The figure shows three views and two pictorial views of one solid part (mm, origin at its lowest corner). Answer the questions. Give positions to 0.01 mm unless a question says otherwise; leave off trailing zeros. Order: outer loops, then holes, each group sorted by start corner. A loop starts at its lowest first (then second) coordinate and runs counter-clockwise, first axis right, second up. Notation, with made-up numbers: (14.25, 35.5) -> (19.25, 35.5) arc R22 cw to (19.25, 45.5) -> close; hole circle Ø4 at (62, 29). An arc over 180 degrees is marked (long way). Use one line per item in the form item = value.
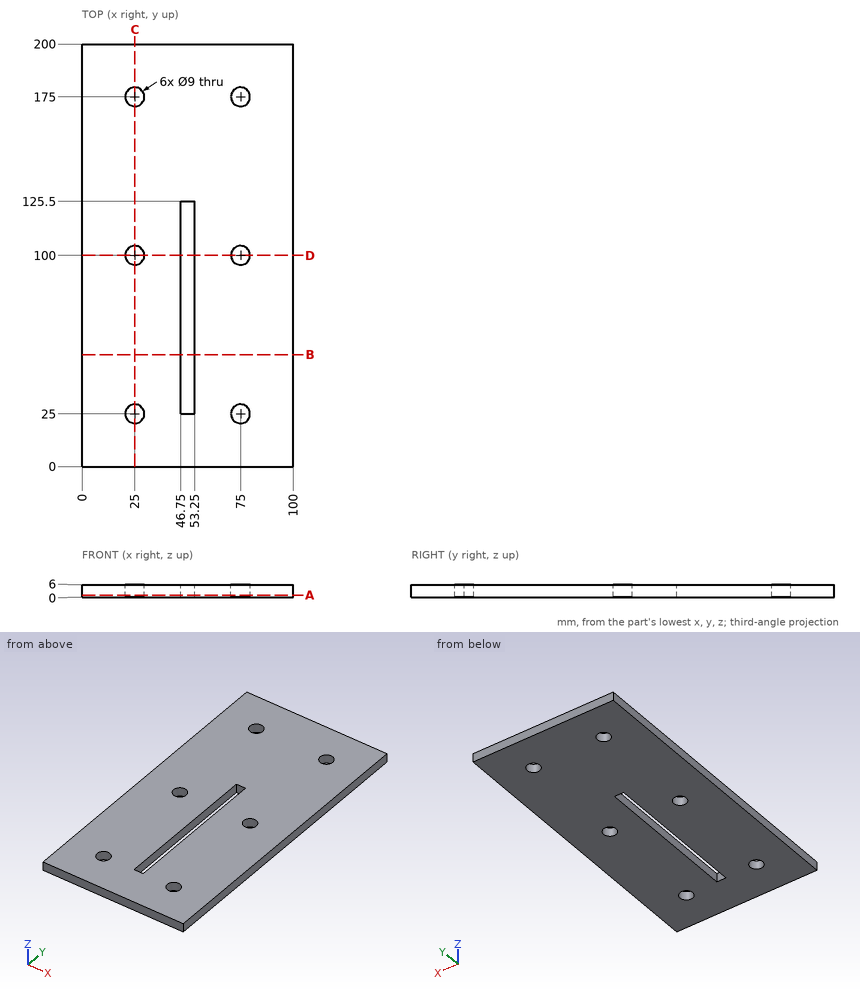
Item 1: The part is cut by section A-A on z = 1. Give the vertices of the cut face in (x, y), and give its area (3 significant figures).
Checks:
outline = (0, 0) -> (100, 0) -> (100, 200) -> (0, 200) -> close; hole circle Ø9 at (25, 25); hole circle Ø9 at (25, 100); hole circle Ø9 at (25, 175); hole (46.75, 25) -> (53.25, 25) -> (53.25, 125.5) -> (46.75, 125.5) -> close; hole circle Ø9 at (75, 25); hole circle Ø9 at (75, 100); hole circle Ø9 at (75, 175)
area = 19,000 mm²
Item 2: Given pin 1 Ø5.5 at (x, y) = (25, 25) entering from +Z, flat-ended and moving along its own axis, determine where the tip first touches the part or whether it passes through.
Checks:
pin_1 = through
Item 3: Straight lines are drawn through the part: L1, parallel to Y at x = 75, z = 2.1; L2, parallel to X at y = 100, z = 2; L3, parallel to X at y = 50.5, z = 3.2. For each, find the intervals that lie inside material, in ascending order. Write a range as from..to.
Checks:
L1 = 0..20.5, 29.5..95.5, 104.5..170.5, 179.5..200
L2 = 0..20.5, 29.5..46.75, 53.25..70.5, 79.5..100
L3 = 0..46.75, 53.25..100
Item 4: The part is cut by section C-C on x = 25. Give the vertices of the cut face in (y, z), and give its area (3 significant figures).
Checks:
outline = (0, 0) -> (20.5, 0) -> (20.5, 6) -> (0, 6) -> close; (29.5, 0) -> (95.5, 0) -> (95.5, 6) -> (29.5, 6) -> close; (104.5, 0) -> (170.5, 0) -> (170.5, 6) -> (104.5, 6) -> close; (179.5, 0) -> (200, 0) -> (200, 6) -> (179.5, 6) -> close
area = 1,040 mm²
Item 5: The part is cut by section B-B on y = 53. Give the vertices of the cut face in (x, z), and give its area (3 significant figures).
Checks:
outline = (0, 0) -> (46.75, 0) -> (46.75, 6) -> (0, 6) -> close; (53.25, 0) -> (100, 0) -> (100, 6) -> (53.25, 6) -> close
area = 561 mm²
Item 6: The part is cut by section D-D on y = 100. Give the vertices of the cut face in (x, z), and give its area (3 significant figures).
Checks:
outline = (0, 0) -> (20.5, 0) -> (20.5, 6) -> (0, 6) -> close; (29.5, 0) -> (46.75, 0) -> (46.75, 6) -> (29.5, 6) -> close; (53.25, 0) -> (70.5, 0) -> (70.5, 6) -> (53.25, 6) -> close; (79.5, 0) -> (100, 0) -> (100, 6) -> (79.5, 6) -> close
area = 453 mm²
